Input: part model. Units: mm. Frame: model coordinates. Coordinates: 2 decimals unless noted, no trailing zeros. Write each loop counter-clockwise with the first axis right and the second up, starting at its lowest first coordinate (ties: lowest second). Pieces come first, ordered by that corner, then holes. Notation, with made-up numbers: M 40,56 L 94,56 A21 cw 94,87 Z; hole C 58,88 d7. An arc over 180 degrees is marked long. Use CSV: the item, a comma, the result in double quotes.
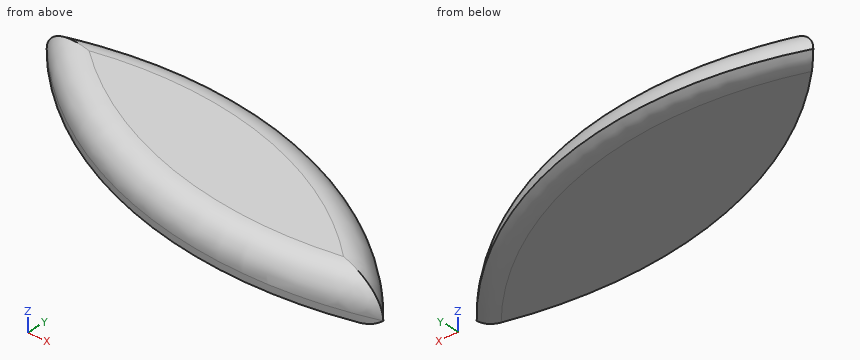
```python
from build123d import *

# Parameters (mm, degrees)
F1_DEPTH    = 6.35
F2_R        = 5.08
F3_T2_ANGLE = 84.7300035824


# Not quite as in the source:
# - a fillet or chamfer that OpenCascade refuses, or shapes differently, is made with other operations: its cross-section is extruded or revolved along the edge and cut away or added


with BuildPart() as f1:
    # F0 (on Top) → F1 (new body)
    with BuildSketch(Plane.XY):
        with BuildLine():
            ThreePointArc((-58.4820285439, 30.5738802999), (-95.0022427224, 52.9656761429), (-137.7363353968, 49.9797277153))
            ThreePointArc((-137.7363353968, 49.9797277153), (-100.9651889281, 28.6127500264), (-58.4820285439, 30.5738802999))
        make_face()
    extrude(amount=F1_DEPTH)

    # F2
    f2_edges = [f1.edges().sort_by_distance(p)[0] for p in [
        (-100.965189, 28.61275, 6.35),
        (-95.002243, 52.965676, 6.35),
    ]]
    fillet(f2_edges, radius=F2_R)

    # F3: fillet of radius 5.08 on 2 edges, made by hand

    # F3_s1 → F3_t2 (revolve, cut)
    with BuildSketch(Plane(origin=(-27.6470070166, 41.1795425882, 0), x_dir=(0, 0, 1), z_dir=(0.557404804, -0.8302408593, 0))):
        with BuildLine():
            ThreePointArc((1.27, 31.0101609977), (0.3280951188, 32.5742139386), (0, 34.3702651628))
            Line((0, 34.3702651628), (0, 31.0101609977))
            Line((0, 31.0101609977), (1.27, 31.0101609977))
        make_face()
    revolve(axis=Axis((-111.7067534455, -15.2562566767, 0), (0, 0, 1)), revolution_arc=F3_T2_ANGLE, mode=Mode.SUBTRACT)


solid = f1.part
```
1. Section A-A (z = 2.75). Return loops of the section in (x, y).
Resolved:
outline,"M -137.35,49.9 A75.09 ccw -58.86,30.68 A70.02 ccw Z"
2. Material intervals for line 1 (X direction, y = 41, z = 3); line 2 (Z direction, x = -118, y = 53.5); line 3 (Y direction, x = -132, z = 4.75), sorted ascending. Write a range as [from, to].
Resolved:
line 1,"x = [-127.03, -70.16]"
line 2,"z = [0.49, 4.54]"
line 3,"y = [46.35, 50.54]"
3. Contact query for flat-ended pins moving along their axis: pin 1 Ø3 at (y, z) = (37.5, 5.5) entering from -X; pin 2 Ø1 at (x, z) = (-75, 3) entering from +Y; pin 3 Ø6 at (x, y) = (-67.5, 40) entering from +Z. Output: stop coordinate, or through.
Resolved:
pin 1,"stops at x = -121.93"
pin 2,"stops at y = 44.63"
pin 3,"stops at z = 5.63"
